Could you check a few things on this model? Use its own coordinates, in mm. Give positions to 0.01 mm unless a question says otherwise; leave off trailing zeros. Loops run counter-clockwise (first coordinate to the right, second up) from the corner with the lowest first, then second, coordinate; pieces in that order, holes last. Notation, with made-up numbers: M 4.5,15 L 30.5,15 A17 ccw 30.5,37 Z; hole C 80.25,-30.5 d1. An arc over 180 degrees is marked long. Use CSV: the item, a comma, the result in double quotes.
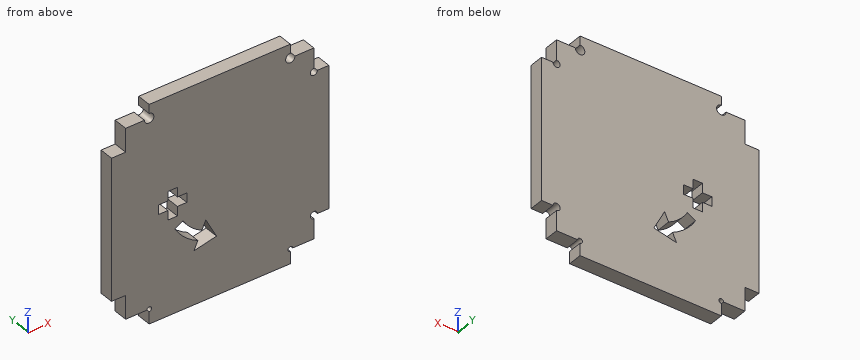
```python
from build123d import *

# Parameters (mm, degrees)
BOSS_EXTRUDE1_DEPTH = 3
SKETCH4_R           = 0.5
SKETCH4_R_2         = 0.75
SKETCH4_R_3         = 1
CUT_EXTRUDE1_DEPTH  = 33.876283245


with BuildPart() as part:
    # Sketch1 → Boss-Extrude1 (new body)
    with BuildSketch(Plane(origin=(0, 0, 0), x_dir=(1, 0, 0), z_dir=(0, 1, 0))):
        Polygon((-20, -20), (-20, -15), (-23, -15), (-23, 15), (-20, 15), (-20, 20), (-15, 20), (-15, 23.1), (15, 23.1), (15, 20), (20, 20), (20, 15), (23.2, 15), (23.2, -15), (20, -15), (20, -20), (15, -20), (15, -22.9), (-15, -22.9), (-15, -20), align=None)
        Polygon((-13, -1), (-11, -1), (-11, -3), (-9, -3), (-9, -1), (-7, -1), (-7, 1), (-9, 1), (-9, 3), (-11, 3), (-11, 1), (-13, 1), align=None, mode=Mode.SUBTRACT)
        with BuildLine():
            Line((-9.526279442, 5.5), (-7.794228634, 4.5))
            ThreePointArc((-7.794228634, 4.5), (-6.080311869, 6.635496031), (-3.803564356, 8.156770083))
            Line((-3.803564356, 8.156770083), (-2.958327832, 6.344154509))
            Line((-2.958327832, 6.344154509), (-0.682812706, 10.715378396))
            Line((-0.682812706, 10.715378396), (-5.494037403, 11.782001231))
            Line((-5.494037403, 11.782001231), (-4.648800879, 9.969385657))
            ThreePointArc((-4.648800879, 9.969385657), (-7.431492284, 8.110050705), (-9.526279442, 5.5))
        make_face(mode=Mode.SUBTRACT)
    extrude(amount=BOSS_EXTRUDE1_DEPTH)

    # Sketch4 → Cut-Extrude1 (cut, through all)
    with BuildSketch(Plane(origin=(0, 3, 0), x_dir=(1, 0, 0), z_dir=(0, 1, 0))):
        with Locations((-15, 20)):
            Circle(SKETCH4_R)
        with Locations((15, 20)):
            Circle(SKETCH4_R)
        with Locations((20, 15)):
            Circle(SKETCH4_R_2)
        with Locations((20, -15)):
            Circle(SKETCH4_R_2)
        with Locations((15, -20)):
            Circle(SKETCH4_R_3)
        with Locations((-15, -20)):
            Circle(SKETCH4_R_3)
    extrude(amount=-CUT_EXTRUDE1_DEPTH, mode=Mode.SUBTRACT)


solid = part.part
```
1. Please list where these lines run through material, in increasing order: line 1 (Z direction, x = -20.5, y = 2.7); line 2 (Z direction, x = 17.5, y = 1.2); line 3 (Z direction, x = -4, y = 2.15).
Outcome:
line 1,"-15 to 15"
line 2,"-20 to 20"
line 3,"-23.1 to -11.45, -8.06 to 22.9"
2. I want a section at A-A, the plane z = 18. List the corners of the cut face in (x, y) for me, then the cut area to 3 significant figures.
Outcome:
outline,"M -20,0 L 20,0 L 20,3 L -20,3 Z"
area,"120 mm2"
3. I'm going to push flat-ended pins straight in: pin 1 Ø0.9 at (y, z) = (1, 18.5) entering from +X; pin 2 Ø1.3 at (y, z) = (2, -21) entering from -X; pin 3 Ø0.7 at (x, y) = (21.5, 2) entering from +Z. Where does each tip first touch, or does it pass through?
Outcome:
pin 1,"x = 20"
pin 2,"x = -15"
pin 3,"z = 15"
4. I want a section at B-B, the plane y = 1.2. Give the number of separate pieces and of enclosed holes in the cut face, then the cut area to 3 significant figures.
Outcome:
separate pieces,"1"
enclosed holes,"2"
area,"1,910 mm2"
